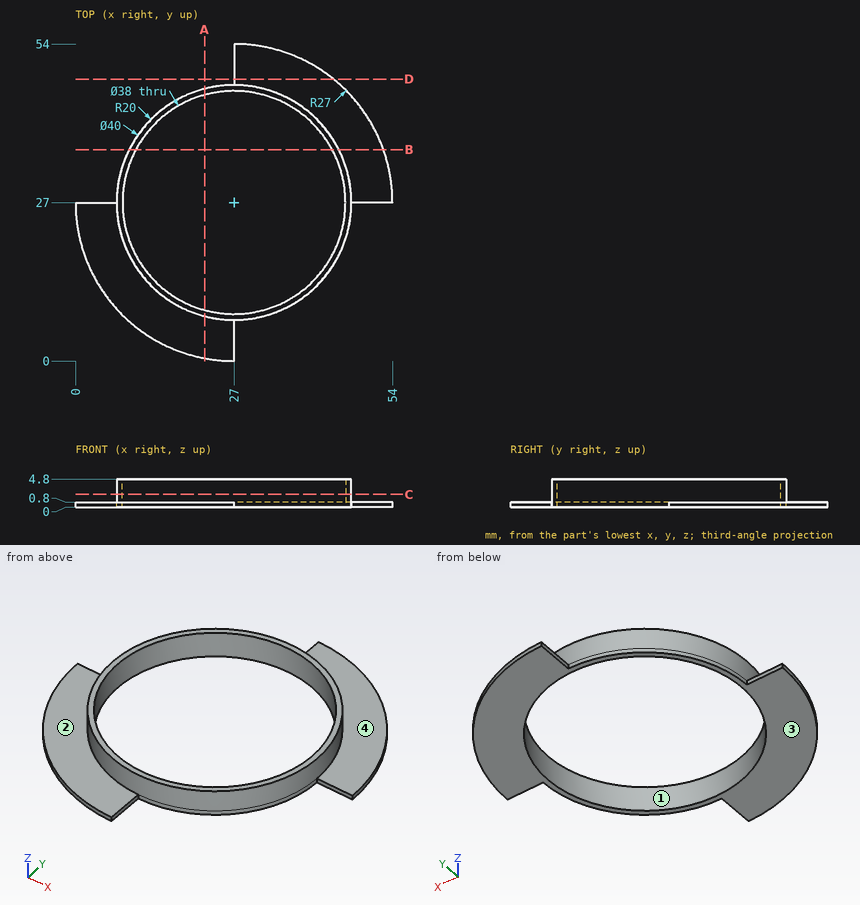
Job drawing, mm, ordinate dimensions from the low corner. One solid piece. A direction names the side the tool comes from. Round coordinates to 2 decimals unless told otherwise and drop trailing zeros. Order: outer loops, then holes, each group sorted by start corner. A loop starts at its lowest first (then second) coordinate and runs counter-clockwise, first axis right, second up. Notation, with made-up numbers: (53.5, -4.75) -> (111.5, -4.75) arc R22 ccw to (111.5, 1.25) -> close; hole circle Ø11 at (37, 86.25). An arc over 180 degrees is marked (long way). Answer in a Markdown table with one row per item.
1) Band-saw the part on D-D on y = 48. Give the cut face in (x, z).
Values:
| item | result |
|---|---|
| outline | (27, 0) -> (43.97, 0) -> (43.97, 0.8) -> (27, 0.8) -> close |
2) Wall check: L1, parallel to Y at x = 27, z = 1; L2, parallel to Z at x = 52, y = 33; L3, parallel to X at y = 13, z = 1.95. Give the ranges that are in metal, low to high.
Values:
| item | result |
|---|---|
| L1 | 7 to 8, 46 to 47 |
| L2 | 0 to 0.8 |
| L3 | 12.72 to 14.15, 39.85 to 41.28 |
3) Which spindle directions (+Z, -Z, +X, -X, +Y, -Y) get a long thin tool onto all of the face, cutting with end or side? Do the marked faces 3 and 4. Say none if no direction does.
Values:
| item | result |
|---|---|
| face 3 | -Z, +X, -X, +Y, -Y |
| face 4 | +Z, +X, +Y |
4) Mould opens along Y. For the marked faces 1 and 2 say: released by +Y, released by -Y, zero draft, split by the parting line, or undercut.
Values:
| item | result |
|---|---|
| face 1 | undercut |
| face 2 | zero draft |
5) Band-saw the part on B-B on y = 36. Give the cut face in (x, z), and give its area (3 significant figures).
Values:
| item | result |
|---|---|
| outline | (9.14, 0) -> (10.27, 0) -> (10.27, 4.8) -> (9.14, 4.8) -> close; (43.73, 0) -> (52.46, 0) -> (52.46, 0.8) -> (44.86, 0.8) -> (44.86, 4.8) -> (43.73, 4.8) -> close |
| area | 16.9 mm2 |
6) Band-saw the part on C-C on z = 2.2. Give the cut face in (x, y).
Values:
| item | result |
|---|---|
| outline | circle Ø40 at (27, 27); hole circle Ø38 at (27, 27) |
7) Band-saw the part on A-A on x = 22. Give the cut face in (y, z), and give its area (3 significant figures).
Values:
| item | result |
|---|---|
| outline | (0.47, 0) -> (8.67, 0) -> (8.67, 4.8) -> (7.64, 4.8) -> (7.64, 0.8) -> (0.47, 0.8) -> close; (45.33, 0) -> (46.36, 0) -> (46.36, 4.8) -> (45.33, 4.8) -> close |
| area | 15.7 mm2 |
8) Pin check, flat tips, straight feed: P1, Ø0.9, axis at x = 2.5, z = 0.5, coming from the +Y side; P2, Ø1, axis at y = 37, z = 3.5, coming from the -X side; P3, Ø0.9, axis at y = 5, z = 0, coming from the +X side. Stop position of each tip, or through.
Values:
| item | result |
|---|---|
| P1 | y = 27 |
| P2 | x = 9.4 |
| P3 | x = 27 |
